Can you work these out from the model? Positions are in its coordinate system, mm. A direction names the side the tool comes from. Round coordinates to 2 decimals unless told otherwise and drop trailing zeros. Loops run counter-clockwise (first coordinate to the right, second up) from the corner with the lowest first, then second, coordinate; pieces in that order, holes last. Notation, with made-up numbers: (56.25, 1.5) - (64.25, 1.5) arc R12 ccw to (64.25, 14.5) - close; hole circle Ø11 at (5, -15). An arc over 180 degrees is marked (long way). Answer as CSV lines item,"result".
```python
from build123d import *

# Parameters (mm, degrees)
SKETCH1_W           = 36.4
SKETCH1_H           = 75.6
SKETCH1_W_2         = 33.2
SKETCH1_H_2         = 72.4
BOSS_EXTRUDE1_DEPTH = 5.2
SKETCH2_W           = 36.4
SKETCH2_H           = 75.6
BOSS_EXTRUDE2_DEPTH = 1.6
BOSS_EXTRUDE3_START = 5.2
SKETCH2_2_W         = 36.4
SKETCH2_2_H         = 75.6
BOSS_EXTRUDE3_DEPTH = 1.6
CUT_EXTRUDE1_START  = -1.6
CUT_EXTRUDE1_DEPTH  = 5.2
BOSS_EXTRUDE4_START = -1.6
BOSS_EXTRUDE4_DEPTH = 33.2
CUT_EXTRUDE2_DEPTH  = 2
FILLET1_R           = 7


with BuildPart() as part:
    # Sketch1 → Boss-Extrude1 (new body)
    with BuildSketch(Plane(origin=(0, 0, 0), x_dir=(1, 0, 0), z_dir=(0, 1, 0))):
        with Locations((16.6, 36.2)):
            Rectangle(SKETCH1_W, SKETCH1_H)
        with Locations((16.6, 36.2)):
            Rectangle(SKETCH1_W_2, SKETCH1_H_2, mode=Mode.SUBTRACT)
    extrude(amount=BOSS_EXTRUDE1_DEPTH)

    # Sketch2 → Boss-Extrude2 (add)
    with BuildSketch(Plane(origin=(0, 0, 0), x_dir=(1, 0, 0), z_dir=(0, 1, 0))):
        with Locations((16.6, 36.2)):
            Rectangle(SKETCH2_W, SKETCH2_H)
    extrude(amount=-BOSS_EXTRUDE2_DEPTH)

    # Sketch2<2> → Boss-Extrude3 (add)
    with BuildSketch(Plane(origin=(0, 0, 0), x_dir=(1, 0, 0), z_dir=(0, 1, 0)).offset(BOSS_EXTRUDE3_START)):
        with Locations((16.6, 36.2)):
            Rectangle(SKETCH2_2_W, SKETCH2_2_H)
    extrude(amount=BOSS_EXTRUDE3_DEPTH)

    # Sketch3 → Cut-Extrude1 (cut)
    with BuildSketch(Plane(origin=(0, 6.8, 0), x_dir=(1, 0, 0), z_dir=(0, 1, 0)).offset(CUT_EXTRUDE1_START)):
        with BuildLine():
            Line((0, 0), (33.2, 0))
            ThreePointArc((33.2, 0), (32.4, -0.8), (33.2, -1.6))
            Line((33.2, -1.6), (0, -1.6))
            ThreePointArc((0, -1.6), (0.8, -0.8), (0, 0))
        make_face()
    extrude(amount=-CUT_EXTRUDE1_DEPTH, mode=Mode.SUBTRACT)

    # Sketch4 → Boss-Extrude4 (add)
    with BuildSketch(Plane(origin=(34.8, 0, 0), x_dir=(0, 0, -1), z_dir=(1, 0, 0)).offset(BOSS_EXTRUDE4_START)):
        with BuildLine():
            Line((1.4, 6.8), (1.4, 8.8))
            ThreePointArc((1.4, 8.8), (2.571572875, 11.628427125), (5.4, 12.8))
            Line((5.4, 12.8), (41.4, 12.8))
            Line((41.4, 12.8), (41.4, 15.8))
            Line((41.4, 15.8), (-1.6, 15.8))
            Line((-1.6, 15.8), (-1.6, 6.8))
            Line((-1.6, 6.8), (1.4, 6.8))
        make_face()
    extrude(amount=-BOSS_EXTRUDE4_DEPTH)

    # Sketch5 → Cut-Extrude2 (cut)
    with BuildSketch(Plane.XZ.offset(1.6)):
        with BuildLine():
            Line((4.4, 1.6), (28.8, 1.6))
            Line((28.8, 1.6), (28.8, -8.4))
            ThreePointArc((28.8, -8.4), (16.6, -20.6), (4.4, -8.4))
            Line((4.4, -8.4), (4.4, 1.6))
        make_face()
    extrude(amount=-CUT_EXTRUDE2_DEPTH, mode=Mode.SUBTRACT)

    # Fillet1
    fillet1_edges = [part.edges().sort_by_distance(p)[0] for p in [
        (16.6, 15.8, 1.6),
    ]]
    fillet(fillet1_edges, radius=FILLET1_R)


solid = part.part
```
Q1. Imagine slicing it at B-B (x = 16.6). Write out the boundary of the cut face in (y, z), then the cut area to 3 significant figures.
Checks:
outline,"(-1.6, -74) - (6.8, -74) - (6.8, -1.4) - (8.8, -1.4) arc R4 cw to (12.8, -5.4) - (12.8, -41.4) - (15.8, -41.4) - (15.8, -5.4) arc R7 ccw to (8.8, 1.6) - (5.2, 1.6) - (5.2, -72.4) - (0, -72.4) - (0, -20.6) - (-1.6, -20.6) - close"
area,"355 mm²"
Q2. We'd pull the mould along Z, two halves only. Please class faces 5 (the flat face through (0, 3, -36)), 6 (the flat face through (16, 6, 1.6)), 7 (the flat face through (-1.6, 3, -36)): pulls with the +Z half, pulls with the -Z half, needs draft (parallel to the pull), parting line crosses it, or undercut.
Checks:
face 5,"undercut"
face 6,"pulls with the +Z half"
face 7,"needs draft"
Q3. Imagine slicing it at D-D (x = 5.5). Write out the boundary of the cut face in (y, z).
Checks:
outline,"(-1.6, -74) - (6.8, -74) - (6.8, -1.4) - (8.8, -1.4) arc R4 cw to (12.8, -5.4) - (12.8, -41.4) - (15.8, -41.4) - (15.8, -5.4) arc R7 ccw to (8.8, 1.6) - (5.2, 1.6) - (5.2, -72.4) - (0, -72.4) - (0, -13.46) - (-1.6, -13.46) - close"
Q4. Imagine slicing it at A-A (z = -37). Write out the boundary of the cut face in (x, y).
Checks:
outline,"(-1.6, -1.6) - (34.8, -1.6) - (34.8, 6.8) - (-1.6, 6.8) - close; (0, 12.8) - (33.2, 12.8) - (33.2, 15.8) - (0, 15.8) - close; hole (0, 0) - (33.2, 0) - (33.2, 5.2) - (0, 5.2) - close"
Q5. I'm going to push flat-ended pins straight in: pin 1 Ø1.6 at (x, y) = (8.5, 3.5) entering from +Z; pin 2 Ø2.5 at (x, y) = (16.5, 15) entering from -Z; pin 3 Ø7 at (y, z) = (10.5, -17) entering from -X. Where does each tip first touch, or does it pass through?
Checks:
pin 1,"z = -72.4"
pin 2,"z = -41.4"
pin 3,"x = 0"
Q6. Imagine slicing it at C-C (y = 1). Write out the boundary of the cut face in (x, z).
Checks:
outline,"(-1.6, -74) - (34.8, -74) - (34.8, 1.6) - (33.2, 1.6) arc R0.8 ccw to (33.2, 0) - (33.2, -72.4) - (0, -72.4) - (0, 0) arc R0.8 ccw to (0, 1.6) - (-1.6, 1.6) - close"
Q7. On a 3-axis mill with a long thin cutter (end or side, diameter ignored), from which of +Z, -Z, +X, -X, +Y, -Y can I reach the whole of each face in a straight line? I mean faces 1 (the cylindrical face through (16.868, -0.811, -20.597)), 2 (the flat face through (33.2, 3, -36)), 3 (the flat face through (33.2, 13, -15)), 4 (the flat face through (17, 14, -41.4)). Say none if no direction works.
Checks:
face 1,"+Z, -Y"
face 2,"none"
face 3,"+Z, -Z, +X, +Y"
face 4,"-Z, +X, -X, +Y"
Q8. If I drill on line 1 along Y through (x, z) = (32.5, -37.5); line 2 along Y through (x, z) = (15, -64.5); line 3 along X through (y, z) = (1, -12.5), over which ranges is the centre line in solid material (lowest first)? Write a range as [from, to].
Checks:
line 1,"[-1.6, 0], [5.2, 6.8], [12.8, 15.8]"
line 2,"[-1.6, 0], [5.2, 6.8]"
line 3,"[-1.6, 0], [33.2, 34.8]"
